Geometry check sheet. Reference: the model listing, model coordinates, mm. A direction names the side the tool comes from. Round coordinates to 2 decimals unless told otherwise and drop trailing zeros. Write each loop counter-clockwise with the first axis right and the second up, starting at its lowest first coordinate (ties: lowest second). Pieces come first, ordered by that corner, then holes.
Autodesk Inventor part; units mm, degrees
ref_plane "Flange Pattern Plane" through (19.05, 7.9375, -4.5466) normal (0, 1, 0) x (1, 0, 0)
ref_plane "YZ Plane" through (0, 0, 0) normal (1, 0, 0) x (0, 1, 0)
ref_plane "XZ Plane" through (0, 0, 0) normal (0, 1, 0) x (-1, 0, 0)
sketch "Sketch1" plane through (0, 0, 0) normal (0, 1, 0) x (-1, 0, 0)
  line L0 (-19.05, 0) -> (19.05, 0)
  line L1 (19.05, 0) -> (19.05, -12.7)
  line L2 (19.05, -12.7) -> (-19.05, -12.7)
  line L3 (-19.05, -12.7) -> (-19.05, 0)
  line L4 (19.05, 0) -> (-19.05, -12.7) construction
  point P0 (0, 0)
  point P1 (0, 0)
  dimension "d0" = 38.1
  dimension "d1" = 12.7
extrude "Plate1" add sketch "Sketch1" along normal blind 1.5875
sketch "Sketch2" plane through (17.4625, 0, -12.7) normal (1, 0, 0) x (0, 1, 0)
  line L0 (0, 12.7) -> (0, 0)
  line L1 (0, 0) -> (14.2875, 0)
  line L2 (14.2875, 0) -> (14.2875, 12.7)
  line L3 (14.2875, 12.7) -> (0, 12.7)
edge flange "Flanges" height 12.7 angle 90 thickness 1.5875 bend radius 0.7937 thickness toward (1, 0, 0) relief tear relief width 1.5875 relief depth 0.7937 corner gap 1.5875 corner form 0 edges at (19.05, 1.5875, -6.35) (-19.05, 1.5875, -6.35) wall of the first edge with corners at (17.4625, 0, 0) (17.4625, 0, -12.7) (17.4625, 14.2875, -12.7) (17.4625, 14.2875, 0)
bend "Bend1"
corner "Corner1"
sketch "Sketch3" plane through (19.05, 2.3813, -12.7) normal (1, 0, 0) x (0, 0, -1)
  line L0 (-8.1534, 7.8676) -> (-4.5466, 7.8676)
  line L1 (-4.0386, 7.3596) -> (-4.0386, 3.7529)
  line L2 (-4.5466, 3.2449) -> (-8.1534, 3.2449)
  line L3 (-8.6614, 3.7529) -> (-8.6614, 7.3596)
  arc A0 (-8.1534, 7.8676) -> (-8.6614, 7.3596) centre (-8.1534, 7.3596) ccw
  arc A1 (-4.0386, 7.3596) -> (-4.5466, 7.8676) centre (-4.5466, 7.3596) ccw
  arc A2 (-4.5466, 3.2449) -> (-4.0386, 3.7529) centre (-4.5466, 3.7529) ccw
  arc A3 (-8.6614, 3.7529) -> (-8.1534, 3.2449) centre (-8.1534, 3.7529) ccw
  line L4 (-12.7, 0) -> (-12.7, 11.9063) construction
  line L5 (-12.7, 11.9063) -> (0, 11.9063) construction
  line L6 (-8.1534, 7.3596) -> (-4.5466, 3.7529) construction
  point P0 (-12.7, -2.3812)
  point P1 (-4.0386, 3.2449)
  point P2 (-8.6614, 3.2449)
  point P3 (-6.35, 5.5563)
  dimension "d16" = 4.6228
  dimension "d17" = 0.508
  dimension "d20" = 6.35
  dimension "d21" = 6.35
extrude "Flange Stamp" cut sketch "Sketch3" against normal blind 1.5875
sketch "Sketch7" plane through (19.05, 2.3813, 0) normal (1, 0, 0) x (0, 0, -1)
  arc A0 (4.5466, 7.8676) -> (4.0386, 7.3596) centre (4.5466, 7.3596) ccw construction
  arc A1 (8.1534, 3.2449) -> (8.6614, 3.7529) centre (8.1534, 3.7529) ccw construction
  circle A2 centre (6.35, 5.5563) radius 2.1844
  line L0 (4.5466, 7.3596) -> (8.1534, 3.7529) construction
  point P0 (0, -2.3812)
  dimension "d46" = 4.3688
surface extrude "Flange Circle" sketch "Sketch7" against normal up to surface (1.5875 mm away) shown yes curves A2
ref_plane "Flange Pattern Plane" through (19.05, 7.9375, -4.5466) normal (0, 1, 0) x (1, 0, 0)
feature "Flange Pattern" [suppressed]
sketch "Sketch8" plane through (0, 0, 0) normal (0, -1, 0) x (1, 0, 0)
  line L0 (16.6687, 0) -> (-16.6687, 0) construction
  line L1 (14.5034, -4.0386) -> (10.8966, -4.0386)
  line L2 (10.3886, -4.5466) -> (10.3886, -8.1534)
  line L3 (10.8966, -8.6614) -> (14.5034, -8.6614)
  line L4 (15.0114, -8.1534) -> (15.0114, -4.5466)
  arc A0 (15.0114, -4.5466) -> (14.5034, -4.0386) centre (14.5034, -4.5466) ccw
  arc A1 (14.5034, -8.6614) -> (15.0114, -8.1534) centre (14.5034, -8.1534) ccw
  arc A2 (10.3886, -8.1534) -> (10.8966, -8.6614) centre (10.8966, -8.1534) ccw
  arc A3 (10.8966, -4.0386) -> (10.3886, -4.5466) centre (10.8966, -4.5466) ccw
  line L5 (14.5034, -4.5466) -> (10.8966, -8.1534) construction
  line L6 (19.05, 0) -> (19.05, -12.7) construction
  point P0 (0, 0)
  point P1 (10.3886, -8.6614)
  point P2 (15.0114, -8.6614)
  point P3 (12.7, -6.35)
  dimension "d49" = 4.6228
  dimension "d50" = 0.508
  dimension "d51" = 6.35
  dimension "d52" = 6.35
extrude "Body Stamp" cut sketch "Sketch8" against normal blind 1.5875
sketch "Sketch9" plane through (0, 0, 0) normal (0, -1, 0) x (1, 0, 0)
  arc A0 (15.0114, -4.5466) -> (14.5034, -4.0386) centre (14.5034, -4.5466) ccw construction
  arc A1 (10.3886, -8.1534) -> (10.8966, -8.6614) centre (10.8966, -8.1534) ccw construction
  line L0 (14.5034, -4.5466) -> (10.8966, -8.1534) construction
  circle A2 centre (12.7, -6.35) radius 2.1844
  point P0 (0, 0)
  dimension "d55" = 4.3688
surface extrude "Body Circle" sketch "Sketch9" against normal up to surface (1.5875 mm away) shown yes curves A2
feature "Body Pattern" [suppressed]
sketch "Arc Length" plane through (17.4625, 2.3813, 0) normal (0, 0, 1) x (1, 0, 0)
  line L0 (0, 0) -> (1.5875, 0) construction
  arc A0 (-0.7938, -0.7938) -> (0, 0) centre (-0.7937, 0) ccw construction
  line L1 (-0.7938, -2.3813) -> (-0.7938, -0.7938) construction
  arc A1 (-0.7938, -2.3813) -> (1.5875, 0) centre (-0.7937, 0) ccw construction
  point P0 (-17.4625, -2.3812)
  dimension "d85" = 3.7405
  dimension "d92" = 1.2468
sketch "Sketch13" plane through (19.05, 14.2875, 0) normal (1, 0, 0) x (0, 0, -1)
  line L0 (0, 0) -> (12.7, 0) construction
  line L1 (62.4078, 0) -> (63.4238, -1.016)
  line L2 (63.4238, -1.016) -> (64.4398, 0)
  line L3 (62.4078, 0) -> (64.4398, 0)
  line L4 (12.7, -11.9063) -> (0, -11.9062) construction
  line L5 (63.4238, -10.8903) -> (61.161, -13.1531)
  line L6 (61.161, -13.1531) -> (63.4238, -15.4159)
  line L7 (63.4238, -15.4159) -> (65.6866, -13.1531)
  line L8 (65.6866, -13.1531) -> (63.4238, -10.8903)
  line L9 (63.4238, -10.8903) -> (63.4238, -15.4159) construction
  line L10 (63.4238, -1.016) -> (63.4238, -10.8903) construction
  line L11 (0, -11.9062) -> (12.7, -11.9063) construction
  point P0 (0, -14.2875)
  dimension "d86" = 4.5256
  dimension "d88" = 1.016
  dimension "d91" = 1.016
  dimension "d102" = 63.4238
feature "Notch" [suppressed]
mirror "Notch Mirror" [suppressed]
pattern_linear "Notch Pattern" [suppressed]
chamfer "End Chamfer" distance 1.016 angle 45 4 edges at (-18.2563, 14.2875, -12.7) (18.2563, 14.2875, -12.7) (-18.2562, 14.2875, 0) (18.2562, 14.2875, 0)
sketch "Sketch14" plane through (-19.05, 2.3813, 431.8) normal (1, 0, 0) x (0, 0, -1)
  line L0 (431.8, 11.9063) -> (444.5, 11.9063) construction
  line L1 (431.8, 0) -> (431.8, 11.9063) construction
  line L2 (431.8, -2.3813) -> (444.5, -2.3813) construction
  line L3 (431.8, 11.9063) -> (444.5, 11.9063)
  line L4 (444.5, 11.9063) -> (444.5, -2.3813)
  line L5 (444.5, -2.3813) -> (431.8, -2.3813)
  line L6 (431.8, -2.3813) -> (431.8, 11.9063)
  point P0 (431.8, -2.3812)
  point P1 (382.0521, -1.9844)
extrude "Half Cut" cut sketch "Sketch14" along normal blind 21.3614
sketch "Flange Pattern Sketch" plane through (19.05, 7.9375, -4.5466) normal (0, 1, 0) x (1, 0, 0)
  line L0 (0, 3.6068) -> (0, 0) construction
  line L1 (-45.8186, -4.5466) -> (8.2118, -4.5466) construction
  line L2 (0, 0) -> (-1.5875, 0) construction
  point P0 (-19.05, -4.5466)
  point P1 (0, 1.8034)
  point P2 (0, 14.5034)
  point P3 (0, 27.2034)
  point P4 (0, 39.9034)
  point P5 (0, 52.6034)
  point P6 (0, 65.3034)
  point P7 (0, 78.0034)
  point P8 (0, 90.7034)
  point P9 (0, 103.4034)
  point P10 (0, 116.1034)
  point P11 (0, 128.8034)
  point P12 (0, 141.5034)
  point P13 (0, 154.2034)
  point P14 (0, 166.9034)
  point P15 (0, 179.6034)
  point P16 (0, 192.3034)
  point P17 (0, 205.0034)
  point P18 (0, 217.7034)
  point P19 (0, 230.4034)
  point P20 (0, 243.1034)
  point P21 (0, 255.8034)
  point P22 (0, 268.5034)
  point P23 (0, 281.2034)
  point P24 (0, 293.9034)
  point P25 (0, 306.6034)
  point P26 (0, 319.3034)
  point P27 (0, 332.0034)
  point P28 (0, 344.7034)
  point P29 (0, 357.4034)
  point P30 (0, 370.1034)
  point P31 (0, 382.8034)
  point P32 (0, 395.5034)
  point P33 (0, 408.2034)
  point P34 (0, 420.9034)
  point P35 (0, 433.6034)
  dimension "d131" = 12.7
  dimension "d134" = 12.7
sketch "Body Pattern Sketch" plane through (0, 0, 0) normal (0, -1, 0) x (1, 0, 0)
  line L0 (16.6687, 0) -> (-16.6687, 0) construction
  line L1 (19.05, 0) -> (19.05, -12.7) construction
  circle A0 centre (12.7, -6.35) radius 2.1844 construction
  point P0 (0, 0)
  point P1 (12.7, -19.05)
  point P2 (12.7, -31.75)
  point P3 (12.7, -44.45)
  point P4 (12.7, -57.15)
  point P5 (12.7, -69.85)
  point P6 (12.7, -82.55)
  point P7 (12.7, -95.25)
  point P8 (12.7, -107.95)
  point P9 (12.7, -120.65)
  point P10 (12.7, -133.35)
  point P11 (12.7, -146.05)
  point P12 (12.7, -158.75)
  point P13 (12.7, -171.45)
  point P14 (12.7, -184.15)
  point P15 (12.7, -196.85)
  point P16 (12.7, -209.55)
  point P17 (12.7, -222.25)
  point P18 (12.7, -234.95)
  point P19 (12.7, -247.65)
  point P20 (12.7, -260.35)
  point P21 (12.7, -273.05)
  point P22 (12.7, -285.75)
  point P23 (12.7, -298.45)
  point P24 (12.7, -311.15)
  point P25 (12.7, -323.85)
  point P26 (12.7, -336.55)
  point P27 (12.7, -349.25)
  point P28 (12.7, -361.95)
  point P29 (12.7, -374.65)
  point P30 (12.7, -387.35)
  point P31 (12.7, -400.05)
  point P32 (12.7, -412.75)
  point P33 (12.7, -425.45)
  point P34 (12.7, -438.15)
  dimension "d62" = 12.7
  dimension "d65" = 12.7
  dimension "d139" = 12.7
equation "\"d1\" = 1.27 * Length"
equation "\"d18\" = Thickness"
equation "\"d53\" = Thickness"
equation "\"d89\" = Thickness"
equation "\"d2\" = Thickness"
equation "\"d3\" = BendReliefWidth"
equation "\"d4\" = BendReliefDepth"
equation "\"d5\" = MinimumRemnant"
equation "\"d6\" = TransitionRadius"
equation "\"d10\" = CornerReliefSize"
equation "\"d11\" = GapSize"
equation "\"d12\" = JacobiRadiusSize"
equation "\"BendRadius\" = Thickness"
equation "\"BendReliefWidth\" = Thickness"
equation "\"BendReliefDepth\" = 0.5 * Thickness"
equation "\"CornerReliefSize\" = 4 * Thickness"
equation "\"MinimumRemnant\" = 2 * Thickness"
equation "\"TransitionRadius\" = BendRadius"
equation "\"JacobiRadiusSize\" = BendRadius"
equation "\"GapSize\" = Thickness"
properties part number "Alu C 1x3x1x35"
1. Section check B-B (z = -5.5). Record the cut outline in (x, y), plus the area to 3 significant figures.
2. Section check A-A (x = 11.5). Record the cut outline in (y, z).
3. Section check C-C (y = 9.25). Record the cut outline in (x, z).
4. Scan lines: line 1 along Y through (x, z) = (5, -3.25); line 2 along X through (y, z) = (5, -9.25); line 3 along Y through (x, z) = (18.5, -7). Record each from-to range of solid material in increasing order.
5. Release check for a two-part mould opening along Y. For faces 5 (the face through (18, 14.288, -6)), 6 (the face through (18, 8, -4.039)), 7 (the face through (14, 1, -12.7)) record: +Y half, -Y half, draft (parallel to the pull), parting line (faces both ways), or undercut.
6. Section check D-D (z = -3). Record the cut outline in (x, y), plus the area to 3 significant figures.
7. Depth check by flat-ended pin: pin 1 Ø0.8 at (x, z) = (18.5, -6.5) entering from -Y; pin 2 Ø5 at (y, z) = (10, -1.5) entering from -X; pin 3 Ø2 at (x, z) = (6.5, -3) entering from -Y; pin 4 Ø1.5 at (x, z) = (9.5, -6.5) entering from +Y. Enter the tip coordinate at first touch or a pass-through.
8. Access from +Z, -Z, +X, -X, +Y, -Y to the whole of each face (thin tool, end or side, straight path). Record for faces 1 (the face through (18.27, 13.79, -12.18)), 2 (the face through (18, 8, -8.661)), 3 (the face through (13, 1, -4.039)), 4 (the face through (10, 1.588, -6)).
Results below:
1. outline: (2.31, 0) - (10.39, 0) - (10.39, 1.59) - (2.31, 1.59) - close; (15.01, 0) - (16.67, 0) arc R2.38 ccw to (19.05, 2.38) - (19.05, 5.63) - (17.46, 5.63) - (17.46, 2.38) arc R0.79 cw to (16.67, 1.59) - (15.01, 1.59) - close; (17.46, 10.25) - (19.05, 10.25) - (19.05, 14.29) - (17.46, 14.29) - close
1. area: 31.0 mm2
2. outline: (0, -12.7) - (1.59, -12.7) - (1.59, -8.66) - (0, -8.66) - close; (0, -4.04) - (1.59, -4.04) - (1.59, 0) - (0, 0) - close
3. outline: (17.46, -12.7) - (19.05, -12.7) - (19.05, -8.66) - (17.46, -8.66) - close; (17.46, -4.04) - (19.05, -4.04) - (19.05, 0) - (17.46, 0) - close
4. line 1: y = 0 to 1.59
4. line 2: x = 17.46 to 19.05
4. line 3: y = 0.86 to 5.63, 10.25 to 14.29
5. face 5: +Y half
5. face 6: undercut
5. face 7: draft
6. outline: (2.31, 0) - (16.67, 0) arc R2.38 ccw to (19.05, 2.38) - (19.05, 14.29) - (17.46, 14.29) - (17.46, 2.38) arc R0.79 cw to (16.67, 1.59) - (2.31, 1.59) - close
6. area: 45.7 mm2
7. pin 1: stops at y = 0.48
7. pin 2: stops at x = 17.46
7. pin 3: stops at y = 0
7. pin 4: stops at y = 1.59
8. face 1: -Z, +X, -X, +Y
8. face 2: +X, -X
8. face 3: +Y, -Y
8. face 4: +Z, -Z, -X, +Y
